from build123d import *

# Parameters (mm, degrees)
F0_R     = 10
F0_R_2   = 8
F0_R_3   = 7
F0_R_4   = 2
F1_DEPTH = 1
F2_DEPTH = 5
F4_DEPTH = 1.5
F6_DEPTH = 1
F8_DEPTH = 9.5


with BuildPart() as f1:
    # F0 (on Top) → F1 (new body)
    with BuildSketch(Plane.XY):
        Circle(F0_R)
        Circle(F0_R_2, mode=Mode.SUBTRACT)
        Circle(F0_R_2)
        Circle(F0_R_3, mode=Mode.SUBTRACT)
        Circle(F0_R_3)
        Circle(F0_R_4, mode=Mode.SUBTRACT)
    extrude(amount=F1_DEPTH)

    # F0 (on Top) → F2 (join)
    with BuildSketch(Plane.XY):
        Circle(F0_R_2)
        Circle(F0_R_3, mode=Mode.SUBTRACT)
    extrude(amount=F2_DEPTH)

    # F3 (on face) → F4 (join)
    with BuildSketch(Plane.XY.offset(1)):
        with BuildLine():
            ThreePointArc((2.6, 6.4992307237), (-2.0663272833, 6.6880708398), (-5.8129166517, 3.9))
            Line((-5.8129166517, 3.9), (2.6, 3.9))
            Line((2.6, 3.9), (2.6, 6.4992307237))
        make_face()
        with BuildLine():
            Line((2.6, 6.4992307237), (2.6, 3.9))
            Line((2.6, 3.9), (5.8129166517, 3.9))
            ThreePointArc((5.8129166517, 3.9), (4.4026459926, 5.4421235069), (2.6, 6.4992307237))
        make_face()
        with BuildLine():
            Line((5.8129166517, 3.9), (2.6, 3.9))
            Line((2.6, 3.9), (2.6, -6.4992307237))
            ThreePointArc((2.6, -6.4992307237), (5.7965506985, -3.9242833741), (7, 0))
            ThreePointArc((7, 0), (6.6966565002, 2.0383306206), (5.8129166517, 3.9))
        make_face()
    extrude(amount=F4_DEPTH)

    # F5 (on Top) → F6 (cut, through all)
    with BuildSketch(Plane.XY):
        with BuildLine():
            ThreePointArc((-3.5, 2), (-4.7803300859, 2.5303300859), (-4.25, 1.25))
            ThreePointArc((-4.25, 1.25), (-3.7196699141, 1.4696699141), (-3.5, 2))
        make_face()
        with BuildLine():
            Line((-4.25, 0), (-3.5, 0))
            ThreePointArc((-3.5, 0), (-3.7196699141, 0.5303300859), (-4.25, 0.75))
            Line((-4.25, 0.75), (-4.25, 0))
        make_face()
        with BuildLine():
            Line((-4.25, -0.75), (-4.25, 0))
            Line((-4.25, 0), (-4.25, 0.75))
            ThreePointArc((-4.25, 0.75), (-5, 0), (-4.25, -0.75))
        make_face()
        with BuildLine():
            ThreePointArc((-4.25, -0.75), (-3.7196699141, -0.5303300859), (-3.5, 0))
            Line((-3.5, 0), (-4.25, 0))
            Line((-4.25, 0), (-4.25, -0.75))
        make_face()
        with BuildLine():
            ThreePointArc((-3.5, -2), (-3.7196699141, -1.4696699141), (-4.25, -1.25))
            ThreePointArc((-4.25, -1.25), (-4.7803300859, -2.5303300859), (-3.5, -2))
        make_face()
    extrude(amount=F6_DEPTH, mode=Mode.SUBTRACT)

    # F7 (on Top) → F8 (join)
    with BuildSketch(Plane.XY):
        with BuildLine():
            Line((-2.5, 3.9), (-2.5, 7.5993420768))
            ThreePointArc((-2.5, 7.5993420768), (-5.0904334607, 6.1715060708), (-6.984983894, 3.9))
            Line((-6.984983894, 3.9), (-2.5, 3.9))
        make_face()
    extrude(amount=F8_DEPTH)


solid = f1.part
Read the model definition and answer for the solid it produces. Units are mm, in the model's axes. A direction names the side the tool comes from. Round coordinates to 2 decimals unless told otherwise and drop trailing zeros. Loops run counter-clockwise (first coordinate to the right, second up) from the corner with the lowest first, then second, coordinate; pieces in that order, holes last. Notation, with made-up numbers: (5.5, -27) - (27.5, -27) arc R12 ccw to (27.5, -17) - close; hole circle Ø3 at (-3, -23). An arc over 180 degrees is marked (long way). One line per question, with ' | ' between items. Start each with the question number.
Q1. For a pull along X with two mould halves and no side action, classify faces 3 (the cylindrical face through (-4.106, -5.669, 3.416)), 4 (the flat face through (-2, -1, 1)), 5 (the cylindrical face through (-2.17, -9.76, 0.49)), 6 (the flat face through (-0.1, 2.4, 0)) as +X half, -X half, draft (parallel to the pull), parting line (faces both ways), or undercut.
Q2. Section B-B on y = -4 is taken. Give the vertices of the cut face in (x, z).
Q3. Flat-ended cylindrical pins translate along their axes: pin 1 (5 mm diameter, centred on x = 2, y = 3, fed in from +Z); pin 2 (1.5 mm diameter, centred on x = 7, y = 3.5, fed in from +Z); pin 3 (3 mm diameter, centred on x = 4.5, z = 4.5, fed in from +Y); pin 4 (8 mm diameter, centred on x = -1, y = 0.5, fed in from -Z). Find the tip coordinate at first contact, or state that the pin passes through.
Q4. Section C-C on x = -4.75 is taken. Give the vertices of the cut face in (y, z).
Q5. For faces 1 (the cylindrical face through (-0.434, -1.952, 0.493)), 2 (the flat face through (0, 8.2, 1)), determine the directions among +Z, -Z, +X, -X, +Y, -Y from which every point of the face is accessible in a straight line to the end or side of a thin tool.
Q6. Find the intervals of material crossed by L1, parallel to Y at x = 0, z = 0.55; L2, parallel to X at y = 0, z = 2.45; L3, parallel to Z at x = -6, y = -7.75, in increasing order.
Q7. Section D-D on y = -1 is taken. Give the vertices of the cut face in (x, z).
Q8. Section A-A on x = 0 is taken. Give the vertices of the cut face in (y, z).
Established:
1) face 3: undercut | face 4: undercut | face 5: parting line | face 6: draft
2) outline: (-9.17, 0) - (9.17, 0) - (9.17, 1) - (6.93, 1) - (6.93, 5) - (5.74, 5) - (5.74, 2.5) - (2.6, 2.5) - (2.6, 1) - (-5.74, 1) - (-5.74, 5) - (-6.93, 5) - (-6.93, 1) - (-9.17, 1) - close
3) pin 1: z = 2.5 | pin 2: z = 5 | pin 3: y = 7.42 | pin 4: z = 0
4) outline: (-8.8, 0) - (-2.56, 0) - (-2.56, 1) - (-5.14, 1) - (-5.14, 5) - (-6.44, 5) - (-6.44, 1) - (-8.8, 1) - close; (-1.44, 0) - (-0.56, 0) - (-0.56, 1) - (-1.44, 1) - close; (0.56, 0) - (1.44, 0) - (1.44, 1) - (0.56, 1) - close; (2.56, 0) - (8.8, 0) - (8.8, 1) - (6.44, 1) - (6.44, 9.5) - (3.9, 9.5) - (3.9, 1) - (2.56, 1) - close
5) face 1: +Z, -Z | face 2: +Z
6) L1: -10 to -2, 2 to 10 | L2: -8 to -7, 2.6 to 8 | L3: 0 to 1
7) outline: (-9.95, 0) - (-1.73, 0) - (-1.73, 1) - (-6.93, 1) - (-6.93, 5) - (-7.94, 5) - (-7.94, 1) - (-9.95, 1) - close; (1.73, 0) - (9.95, 0) - (9.95, 1) - (7.94, 1) - (7.94, 5) - (6.93, 5) - (6.93, 2.5) - (2.6, 2.5) - (2.6, 1) - (1.73, 1) - close
8) outline: (-10, 0) - (-2, 0) - (-2, 1) - (-7, 1) - (-7, 5) - (-8, 5) - (-8, 1) - (-10, 1) - close; (2, 0) - (10, 0) - (10, 1) - (8, 1) - (8, 5) - (7, 5) - (7, 2.5) - (3.9, 2.5) - (3.9, 1) - (2, 1) - close
